```python
from build123d import *

# Parameters (mm, degrees)
BOSS_EXTRUDE1_DEPTH             = 7
F_6_0MM_DOWEL_HOLE1_D           = 6
F_6_0MM_DOWEL_HOLE1_CSINK_D     = 6.05
F_6_0MM_DOWEL_HOLE1_CSINK_ANGLE = 90
BOSS_EXTRUDE2_DEPTH             = 76
BOSS_EXTRUDE2_DEPTH_BACK        = 7
SKETCH5_W                       = 65
SKETCH5_H                       = 47
FILLET1_R                       = 7.5
F_6_0MM_DOWEL_HOLE2_D           = 7
CUT_EXTRUDE1_DEPTH              = 40
BOSS_EXTRUDE3_START             = 27
BOSS_EXTRUDE3_DEPTH             = 27
BOSS_EXTRUDE4_START             = 7.5
BOSS_EXTRUDE4_DEPTH             = 7.5
F_6_0MM_DOWEL_HOLE3_D           = 6
CUT_EXTRUDE2_DEPTH              = 14.5
BOSS_EXTRUDE5_DEPTH             = 1
F_5_0MM_DOWEL_HOLE1_D           = 5
F_5_0MM_DOWEL_HOLE1_DEPTH       = 13
F_5_0MM_DOWEL_HOLE1_TIP         = 1.502151548
BOSS_EXTRUDE6_DEPTH             = 2
CUT_EXTRUDE4_DEPTH              = 11.5
SKETCH27_R                      = 9
CUT_EXTRUDE5_DEPTH              = 30
SKETCH28_R                      = 5
CUT_EXTRUDE6_DEPTH              = 100
SKETCH29_R                      = 18
BOSS_EXTRUDE7_DEPTH             = 47
SKETCH30_R                      = 13.5
CUT_EXTRUDE7_DEPTH              = 37
SKETCH31_R                      = 12
CUT_EXTRUDE8_DEPTH              = 5
SKETCH32_R                      = 5
CUT_EXTRUDE9_DEPTH              = 116.161842639
SKETCH33_R                      = 3.5
CUT_EXTRUDE10_DEPTH             = 10
FILLET4_R                       = 2


with BuildPart() as part:
    # Sketch2 → Boss-Extrude1 (new body)
    with BuildSketch(Plane(origin=(0, 0, 0), x_dir=(1, 0, 0), z_dir=(0, 1, 0))):
        with BuildLine():
            Line((-29, -36.5), (29, -36.5))
            ThreePointArc((29, -36.5), (34.303300859, -34.303300859), (36.5, -29))
            Line((36.5, -29), (36.5, 29))
            ThreePointArc((36.5, 29), (34.303300859, 34.303300859), (29, 36.5))
            Line((29, 36.5), (-29, 36.5))
            ThreePointArc((-29, 36.5), (-34.303300859, 34.303300859), (-36.5, 29))
            Line((-36.5, 29), (-36.5, -29))
            ThreePointArc((-36.5, -29), (-34.303300859, -34.303300859), (-29, -36.5))
        make_face()
    extrude(amount=BOSS_EXTRUDE1_DEPTH)

    # Ø6.0mm Dowel Hole1 (through all)
    with Locations(Plane(origin=(-29, 7, -29), x_dir=(0, 0, 1), z_dir=(0, 1, 0))):
        with Locations((0, 0), (0, 58), (58, 58), (58, 0)):
            CounterSinkHole(F_6_0MM_DOWEL_HOLE1_D / 2, F_6_0MM_DOWEL_HOLE1_CSINK_D / 2, counter_sink_angle=F_6_0MM_DOWEL_HOLE1_CSINK_ANGLE)

    # Sketch5 → Boss-Extrude2 (add, two sides: drawn at the far end of the back side and taken through both)
    with BuildSketch(Plane(origin=(0, 7, 0), x_dir=(1, 0, 0), z_dir=(0, 1, 0)).offset(-BOSS_EXTRUDE2_DEPTH_BACK)):
        with Locations((-14.5, -1)):
            Rectangle(SKETCH5_W, SKETCH5_H)
    extrude(amount=BOSS_EXTRUDE2_DEPTH + BOSS_EXTRUDE2_DEPTH_BACK)

    # Fillet1
    fillet1_edges = [part.edges().sort_by_distance(p)[0] for p in [
        (18, 83, 1),
        (-47, 83, 1),
    ]]
    fillet(fillet1_edges, radius=FILLET1_R)

    # Ø6.0mm Dowel Hole2 (through all)
    with Locations(Plane(origin=(-39.5, 75.5, 24.5), x_dir=(1, 0, 0), z_dir=(0, 0, 1))):
        with Locations((0, 0), (50, 0), (0, -55), (50, -55)):
            Hole(F_6_0MM_DOWEL_HOLE2_D / 2)

    # Sketch9 → Cut-Extrude1 (cut)
    with BuildSketch(Plane.XY.offset(24.5)):
        with BuildLine():
            Line((11, 66.11916848), (11, 51))
            ThreePointArc((11, 51), (11.585786438, 49.585786438), (13, 49))
            ThreePointArc((13, 49), (14.414213562, 48.414213562), (15, 47))
            Line((15, 47), (15, 30))
            ThreePointArc((15, 30), (14.414213562, 28.585786438), (13, 28))
            Line((13, 28), (10.5, 28))
            ThreePointArc((10.5, 28), (5.196699141, 25.803300859), (3, 20.5))
            Line((3, 20.5), (3, 12))
            ThreePointArc((3, 12), (2.414213562, 10.585786438), (1, 10))
            Line((1, 10), (-30, 10))
            ThreePointArc((-30, 10), (-31.414213562, 10.585786438), (-32, 12))
            Line((-32, 12), (-32, 20.5))
            ThreePointArc((-32, 20.5), (-33.793355673, 25.366642634), (-38.315789474, 27.905919621))
            ThreePointArc((-38.315789474, 27.905919621), (-39.521771821, 28.583060151), (-40, 29.88083152))
            Line((-40, 29.88083152), (-40, 66.11916848))
            ThreePointArc((-40, 66.11916848), (-39.521771821, 67.416939849), (-38.315789474, 68.094080379))
            ThreePointArc((-38.315789474, 68.094080379), (-34.196699141, 70.196699141), (-32.094080379, 74.315789474))
            ThreePointArc((-32.094080379, 74.315789474), (-31.416939849, 75.521771821), (-30.11916848, 76))
            Line((-30.11916848, 76), (1.11916848, 76))
            ThreePointArc((1.11916848, 76), (2.416939849, 75.521771821), (3.094080379, 74.315789474))
            ThreePointArc((3.094080379, 74.315789474), (5.196699141, 70.196699141), (9.315789474, 68.094080379))
            ThreePointArc((9.315789474, 68.094080379), (10.521771821, 67.416939849), (11, 66.11916848))
        make_face()
    extrude(amount=-CUT_EXTRUDE1_DEPTH, mode=Mode.SUBTRACT)

    # Sketch11 → Boss-Extrude3 (add)
    with BuildSketch(Plane.XY.offset(-15.5).offset(BOSS_EXTRUDE3_START)):
        with BuildLine():
            Line((-32, 20.5), (-32, 50))
            Line((-32, 50), (-40, 50))
            Line((-40, 50), (-40, 29.88083152))
            ThreePointArc((-40, 29.88083152), (-39.521771821, 28.583060151), (-38.315789474, 27.905919621))
            ThreePointArc((-38.315789474, 27.905919621), (-33.793355673, 25.366642634), (-32, 20.5))
        make_face()
    extrude(amount=-BOSS_EXTRUDE3_DEPTH)

    # Sketch12 → Boss-Extrude4 (add)
    with BuildSketch(Plane.XY.offset(-15.5).offset(BOSS_EXTRUDE4_START)):
        with BuildLine():
            Line((-9.5, 10), (-9.5, 19.5))
            ThreePointArc((-9.5, 19.5), (-11.696699141, 24.803300859), (-17, 27))
            Line((-17, 27), (-32, 27))
            Line((-32, 27), (-32, 12))
            ThreePointArc((-32, 12), (-31.414213562, 10.585786438), (-30, 10))
            Line((-30, 10), (-9.5, 10))
        make_face()
    extrude(amount=-BOSS_EXTRUDE4_DEPTH)

    # Ø6.0mm Dowel Hole3 (through all)
    with Locations(Plane(origin=(-17, 19.5, -8), x_dir=(1, 0, 0), z_dir=(0, 0, 1))):
        with Locations((0, 0)):
            Hole(F_6_0MM_DOWEL_HOLE3_D / 2)

    # Sketch14 → Cut-Extrude2 (cut)
    with BuildSketch(Plane(origin=(0, 0, -22.5), x_dir=(-1, 0, 0), z_dir=(0, 0, -1))):
        with BuildLine():
            Line((-5.832809465, 48), (-5.832809465, 30))
            ThreePointArc((-5.832809465, 30), (2.167190535, 22), (10.167190535, 30))
            Line((10.167190535, 30), (10.167190535, 48))
            ThreePointArc((10.167190535, 48), (2.167190535, 56), (-5.832809465, 48))
        make_face()
    extrude(amount=-CUT_EXTRUDE2_DEPTH, mode=Mode.SUBTRACT)

    # Sketch15 → Boss-Extrude5 (add)
    with BuildSketch(Plane.ZY.offset(47)):
        with BuildLine():
            Line((24.5, 0), (-22.5, 0))
            Line((-22.5, 0), (-22.5, 23))
            ThreePointArc((-22.5, 23), (-21.914213562, 24.414213562), (-20.5, 25))
            Line((-20.5, 25), (22.5, 25))
            ThreePointArc((22.5, 25), (23.914213562, 24.414213562), (24.5, 23))
            Line((24.5, 23), (24.5, 0))
        make_face()
    extrude(amount=BOSS_EXTRUDE5_DEPTH)

    # Ø5.0mm Dowel Hole1
    with Locations(Plane(origin=(-48, 12.5, 18.5), x_dir=(0, 0, -1), z_dir=(-1, 0, 0))):
        with Locations((0, 0), (37, 0)):
            Hole(F_5_0MM_DOWEL_HOLE1_D / 2, depth=F_5_0MM_DOWEL_HOLE1_DEPTH)
            with Locations((0, 0, -(F_5_0MM_DOWEL_HOLE1_DEPTH + F_5_0MM_DOWEL_HOLE1_TIP / 2))):  # 118° drill point
                Cone(0, F_5_0MM_DOWEL_HOLE1_D / 2, F_5_0MM_DOWEL_HOLE1_TIP, mode=Mode.SUBTRACT)

    # Sketch21 → Boss-Extrude6 (add)
    with BuildSketch(Plane(origin=(0, 0, -22.5), x_dir=(-1, 0, 0), z_dir=(0, 0, -1))):
        Polygon((48, 0), (36.5, 0), (36.5, 7), (-18, 7), (-18, 12), (48, 12), align=None)
    extrude(amount=BOSS_EXTRUDE6_DEPTH)

    # Sketch23 → Cut-Extrude4 (cut)
    with BuildSketch(Plane.ZY.offset(48)):
        with BuildLine():
            Line((-22.5, 0), (-24.5, 0))
            Line((-24.5, 0), (-24.5, 2))
            ThreePointArc((-24.5, 2), (-23.914213562, 0.585786438), (-22.5, 0))
        make_face()
        with BuildLine():
            Line((24.5, 0), (22.5, 0))
            ThreePointArc((22.5, 0), (23.914213562, 0.585786438), (24.5, 2))
            Line((24.5, 2), (24.5, 0))
        make_face()
    extrude(amount=-CUT_EXTRUDE4_DEPTH, mode=Mode.SUBTRACT)

    # Sketch27 → Cut-Extrude5 (cut)
    with BuildSketch(Plane.XZ):
        with Locations(Location((0, 0, 0), (0, 0, 270))):
            Circle(SKETCH27_R)
    extrude(amount=-CUT_EXTRUDE5_DEPTH, mode=Mode.SUBTRACT)

    # Sketch28 → Cut-Extrude6 (cut)
    with BuildSketch(Plane.ZY.offset(47)):
        with Locations(Location((-1.5, 33, 0), (0, 0, 323.130102354))):
            Circle(SKETCH28_R)
    extrude(amount=-CUT_EXTRUDE6_DEPTH, mode=Mode.SUBTRACT)

    # Sketch29 → Boss-Extrude7 (add)
    with BuildSketch(Plane(origin=(18, 0, 0), x_dir=(0, 0, -1), z_dir=(1, 0, 0))):
        with Locations((1.5, 33)):
            Circle(SKETCH29_R)
    extrude(amount=BOSS_EXTRUDE7_DEPTH)

    # Sketch30 → Cut-Extrude7 (cut)
    with BuildSketch(Plane(origin=(65, 0, 0), x_dir=(0, 0, -1), z_dir=(1, 0, 0))):
        with Locations((1.5, 33)):
            Circle(SKETCH30_R)
    extrude(amount=-CUT_EXTRUDE7_DEPTH, mode=Mode.SUBTRACT)

    # Sketch31 → Cut-Extrude8 (cut)
    with BuildSketch(Plane(origin=(28, 0, 0), x_dir=(0, 0, -1), z_dir=(1, 0, 0))):
        with Locations((1.5, 33)):
            Circle(SKETCH31_R)
    extrude(amount=-CUT_EXTRUDE8_DEPTH, mode=Mode.SUBTRACT)

    # Sketch32 → Cut-Extrude9 (cut, through all)
    with BuildSketch(Plane(origin=(23, 0, 0), x_dir=(0, 0, -1), z_dir=(1, 0, 0))):
        with Locations(Location((1.5, 33, 0), (0, 0, 216.869897646))):
            Circle(SKETCH32_R)
    extrude(amount=-CUT_EXTRUDE9_DEPTH, mode=Mode.SUBTRACT)

    # Sketch33 → Cut-Extrude10 (cut)
    with BuildSketch(Plane(origin=(0, 83, 0), x_dir=(1, 0, 0), z_dir=(0, 1, 0))):
        with Locations(Location((-14.5, -1, 0), (0, 0, 270))):
            Circle(SKETCH33_R)
    extrude(amount=-CUT_EXTRUDE10_DEPTH, mode=Mode.SUBTRACT)

    # Fillet4
    fillet4_edges = [part.edges().sort_by_distance(p)[0] for p in [
        (34.303300859, 7, -34.303300859),
        (0, 7, -36.5),
        (-34.303300859, 7, -34.303300859),
        (-36.5, 7, -26.75),
        (-34.303300859, 7, 34.303300859),
        (0, 7, 36.5),
        (34.303300859, 7, 34.303300859),
        (-36.5, 7, 26.75),
        (36.5, 7, 0),
    ]]
    fillet(fillet4_edges, radius=FILLET4_R)


solid = part.part
```
Source: CAD feature listing. Evaluate the final solid. Frame: model axes, mm. A direction names the side the tool comes from. Coordinates: 2 decimals unless noted, no trailing zeros. Loops run counter-clockwise (first coordinate to the right, second up) from the corner with the lowest first, then second, coordinate; pieces in that order, holes last. Notation, with made-up numbers: M 88,45.5 L 127,45.5 A15 cw 127,64.5 Z; hole C -24,44 d11. An arc over 180 degrees is marked long. Use a Markdown table: item, result. Add a question column.
Q1. Material intervals for L1, parallel to X at y = 2.5, z = 29; L2, parallel to Y at x = 26.2, z = -1.5, sorted ascending.
Q2. Access query for faces 1 (the cylindrical face through (46.76, 19.82, 1.43)), 2 (the flat face through (-21, 19, -8)), 3 (the flat face through (5.833, 39, -19)), 4 (the cylindrical face through (34.245, 2.465, 34.361)). Directions: +Z, -Z, +X, -X, +Y, -Y. A direction counts if a zero-diameter tool reaches every point of the face in a straight line with its end or side. Return the directions, or none.
Q3. Draft query along Z for faces 5 (the flat face through (-24, 27, -12)), 6 (the flat face through (-15, 47, -22.5)), 7 (the cylindrical face through (29, 3, -26)). Return one class per face: pulls with the +Z half, pulls with the -Z half, needs draft (parallel to the pull), parting line crosses it, or undercut.
Q4. Section query B-B, the plane x = 44. Return loops of the section in (y, z).
Q5. Section query A-A, the plane z = 0. State how many separate pieces and enclosed holes the cut face has, and give its area (3 significant figures).
Q6. First-contact query: pin 1 (9 mm diameter, centred on x = 10.5, y = 75.5, fed in from +Z); pin 2 (3 mm diameter, centred on y = 57, z = 12.5, fed in from -X); pin 3 (20 mm diameter, centred on x = -23, y = 56, fed in from -Z). Flat tips, straight axial feed; report the tip coordinate or a pass-through.
Result:
| question | item | result |
|---|---|---|
| 1 | L1 | x = -36.5 to -32, -26 to 26, 32 to 36.5 |
| 1 | L2 | y = 0 to 7, 15 to 21, 45 to 51 |
| 2 | face 1 | +X |
| 2 | face 2 | +Z |
| 2 | face 3 | +Z, -Z |
| 2 | face 4 | +Z, +X, +Y, -Y |
| 3 | face 5 | needs draft |
| 3 | face 6 | pulls with the -Z half |
| 3 | face 7 | undercut |
| 4 | outline | C 33,-1.5 d36; hole C 33,-1.5 d27 |
| 5 | separate pieces | 4 |
| 5 | enclosed holes | 3 |
| 5 | area | 2,520 mm2 |
| 6 | pin 1 | stops at z = 24.5 |
| 6 | pin 2 | stops at x = -47 |
| 6 | pin 3 | stops at z = -22.5 |
